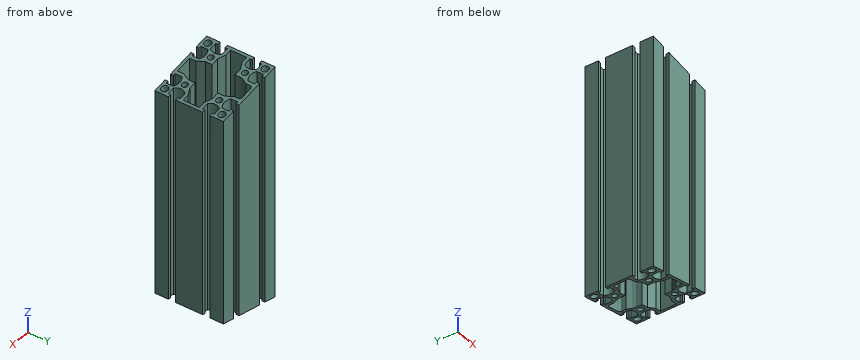
from build123d import *

# Parameters (mm, degrees)
F0_R          = 3
F0_R_2        = 2.5
F1_DEPTH      = 200
F2_R          = 2
F3_R          = 7
F6_DEPTH      = 30
F6_DEPTH_BACK = 30


# Not quite as in the source:
# - a feature names something its author has since deleted; it is built from what else it names


with BuildPart() as f1:
    # F0 (on Top) → F1 (new body)
    with BuildSketch(Plane.XY):
        with BuildLine():
            Line((18.15, -30), (30, -30))
            Line((30, -30), (30, -18.15))
            Line((30, -18.15), (27.5, -18.15))
            Line((27.5, -18.15), (27.5, -20.15))
            Line((27.5, -20.15), (21.5477069044, -20.15))
            ThreePointArc((21.5477069044, -20.15), (19.5, -15), (21.5477069044, -9.85))
            Line((21.5477069044, -9.85), (27.5, -9.85))
            Line((27.5, -9.85), (27.5, -11.85))
            Line((27.5, -11.85), (30, -11.85))
            Line((30, -11.85), (30, 11.85))
            Line((30, 11.85), (27.5, 11.85))
            Line((27.5, 11.85), (27.5, 9.85))
            Line((27.5, 9.85), (21.5477069044, 9.85))
            ThreePointArc((21.5477069044, 9.85), (19.5, 15), (21.5477069044, 20.15))
            Line((21.5477069044, 20.15), (27.5, 20.15))
            Line((27.5, 20.15), (27.5, 18.15))
            Line((27.5, 18.15), (30, 18.15))
            Line((30, 18.15), (30, 30))
            Line((30, 30), (18.15, 30))
            Line((18.15, 30), (18.15, 27.5))
            Line((18.15, 27.5), (20.15, 27.5))
            Line((20.15, 27.5), (20.15, 21.5477069044))
            ThreePointArc((20.15, 21.5477069044), (15, 19.5), (9.85, 21.5477069044))
            Line((9.85, 21.5477069044), (9.85, 27.5))
            Line((9.85, 27.5), (11.85, 27.5))
            Line((11.85, 27.5), (11.85, 30))
            Line((11.85, 30), (-11.85, 30))
            Line((-11.85, 30), (-11.85, 27.5))
            Line((-11.85, 27.5), (-9.85, 27.5))
            Line((-9.85, 27.5), (-9.85, 21.5477069044))
            ThreePointArc((-9.85, 21.5477069044), (-15, 19.5), (-20.15, 21.5477069044))
            Line((-20.15, 21.5477069044), (-20.15, 27.5))
            Line((-20.15, 27.5), (-18.15, 27.5))
            Line((-18.15, 27.5), (-18.15, 30))
            Line((-18.15, 30), (-30, 30))
            Line((-30, 30), (-30, 18.15))
            Line((-30, 18.15), (-27.5, 18.15))
            Line((-27.5, 18.15), (-27.5, 20.15))
            Line((-27.5, 20.15), (-21.5477069044, 20.15))
            ThreePointArc((-21.5477069044, 20.15), (-19.5, 15), (-21.5477069044, 9.85))
            Line((-21.5477069044, 9.85), (-27.5, 9.85))
            Line((-27.5, 9.85), (-27.5, 11.85))
            Line((-27.5, 11.85), (-30, 11.85))
            Line((-30, 11.85), (-30, -11.85))
            Line((-30, -11.85), (-27.5, -11.85))
            Line((-27.5, -11.85), (-27.5, -9.85))
            Line((-27.5, -9.85), (-21.5477069044, -9.85))
            ThreePointArc((-21.5477069044, -9.85), (-19.5, -15), (-21.5477069044, -20.15))
            Line((-21.5477069044, -20.15), (-27.5, -20.15))
            Line((-27.5, -20.15), (-27.5, -18.15))
            Line((-27.5, -18.15), (-30, -18.15))
            Line((-30, -18.15), (-30, -30))
            Line((-30, -30), (-18.15, -30))
            Line((-18.15, -30), (-18.15, -27.5))
            Line((-18.15, -27.5), (-20.15, -27.5))
            Line((-20.15, -27.5), (-20.15, -21.5477069044))
            ThreePointArc((-20.15, -21.5477069044), (-15, -19.5), (-9.85, -21.5477069044))
            Line((-9.85, -21.5477069044), (-9.85, -27.5))
            Line((-9.85, -27.5), (-11.85, -27.5))
            Line((-11.85, -27.5), (-11.85, -30))
            Line((-11.85, -30), (11.85, -30))
            Line((11.85, -30), (11.85, -27.5))
            Line((11.85, -27.5), (9.85, -27.5))
            Line((9.85, -27.5), (9.85, -21.5477069044))
            ThreePointArc((9.85, -21.5477069044), (15, -19.5), (20.15, -21.5477069044))
            Line((20.15, -21.5477069044), (20.15, -27.5))
            Line((20.15, -27.5), (18.15, -27.5))
            Line((18.15, -27.5), (18.15, -30))
        make_face()
        with Locations((-25, -25)):
            Circle(F0_R, mode=Mode.SUBTRACT)
        with Locations((-15, -15)):
            Circle(F0_R_2, mode=Mode.SUBTRACT)
        with Locations((25, -25)):
            Circle(F0_R, mode=Mode.SUBTRACT)
        with Locations((15, -15)):
            Circle(F0_R_2, mode=Mode.SUBTRACT)
        with Locations((-25, 25)):
            Circle(F0_R, mode=Mode.SUBTRACT)
        with Locations((-15, 15)):
            Circle(F0_R_2, mode=Mode.SUBTRACT)
        Polygon((-7, 22), (-7, 27.5), (0, 27.5), (7, 27.5), (7, 22), (10, 16), (10, 10), (16, 10), (22, 7), (27.5, 7), (27.5, 0), (27.5, -7), (22, -7), (16, -10), (10, -10), (10, -16), (7, -22), (7, -27.5), (0, -27.5), (-7, -27.5), (-7, -22), (-10, -16), (-10, -10), (-16, -10), (-22, -7), (-27.5, -7), (-27.5, 0), (-27.5, 7), (-22, 7), (-16, 10), (-10, 10), (-10, 16), align=None, mode=Mode.SUBTRACT)
        with Locations((15, 15)):
            Circle(F0_R_2, mode=Mode.SUBTRACT)
        with Locations((25, 25)):
            Circle(F0_R, mode=Mode.SUBTRACT)
    extrude(amount=F1_DEPTH)

    # F2
    f2_edges = [f1.edges().sort_by_distance(p)[0] for p in [
        (-7, 27.5, 100),
        (7, 27.5, 100),
    ]]
    fillet(f2_edges, radius=F2_R)

    # F3
    f3_edges = [f1.edges().sort_by_distance(p)[0] for p in [
        (-10, 16, 100),
        (10, 16, 100),
    ]]
    fillet(f3_edges, radius=F3_R)

    # F5 (on Front) → F6 (cut, two sides)
    with BuildSketch(Plane.XZ) as f6_sk:
        Polygon((161.6827257777, -158.1931300344), (124.1182914407, 30.656034207), (-30, 0), (7.5644343369, -188.8491642414), align=None)
        Polygon((119.7769204661, 170.2075181713), (153.4553825462, 339.5205806204), (3.6784620801, 369.3130624492), (-30, 200), align=None)
    extrude(amount=F6_DEPTH, mode=Mode.SUBTRACT)
    extrude(f6_sk.sketch, amount=-F6_DEPTH_BACK, mode=Mode.SUBTRACT)


solid = f1.part
Here's how the part is built. I have some questions about the finished solid (model axes, mm). Coordinates: 2 decimals unless noted, no trailing zeros. Loops run counter-clockwise (first coordinate to the right, second up) from the corner with the lowest first, then second, coordinate; pieces in that order, holes last. Notation, with made-up numbers: (-22.5, -27) -> (34.5, -27) arc R12 cw to (34.5, -17) -> close; hole circle Ø2 at (60, -35). An arc over 180 degrees is marked (long way). Use one line per item in the form item = value. Start each with the question number.
(1) Will these pins go through, and if not, where does the flat tip stop? pin 1 (4 mm diameter, centred on x = 12, y = 16.5, fed in from -Z); pin 2 (5 mm diameter, centred on x = 14, y = -19.5, fed in from +Z).
(2) Please list where these lines run through material, in increasing order: line 1 along X through (y, z) = (-25, 55); line 2 along Y through (x, z) = (-15, 158).
(3) If we section it at A-A (x = 24.5): Please give me the cut outline in (y, z).
(4) If we section it at B-B (z = 82): Give the number of separate pieces and of enclosed holes in the cut face, then the cut area to 3 significant figures.
Verdict:
q1.pin_1 = 7.96
q1.pin_2 = 191.75
q2.line_1 = -30 to -28, -22 to -20.15, -9.85 to -7, 7 to 9.85, 20.15 to 22, 28 to 30
q2.line_2 = -19.5 to -17.5, -12.5 to -10, 10 to 12.5, 17.5 to 19.5
q3.outline = (-30, 10.84) -> (-27.96, 10.84) -> (-27.96, 189.16) -> (-30, 189.16) -> close; (-22.04, 10.84) -> (-20.15, 10.84) -> (-20.15, 189.16) -> (-22.04, 189.16) -> close; (-9.85, 10.84) -> (-7, 10.84) -> (-7, 189.16) -> (-9.85, 189.16) -> close; (7, 10.84) -> (9.85, 10.84) -> (9.85, 189.16) -> (7, 189.16) -> close; (20.15, 10.84) -> (22.04, 10.84) -> (22.04, 189.16) -> (20.15, 189.16) -> close; (27.96, 10.84) -> (30, 10.84) -> (30, 189.16) -> (27.96, 189.16) -> close
q4.separate_pieces = 1
q4.enclosed_holes = 9
q4.area = 1,080 mm²
